```python
from build123d import *

# Parameters (mm, degrees)
SKETCH1_R                 = 10
BOSS_EXTRUDE2_DEPTH       = 35
SHELL1_T                  = -2.5
SHELL1_THICKNESS_2_FACE_R = 7.5
SHELL1_THICKNESS_2_DEPTH  = 27.5
SKETCH2_R                 = 1
BOSS_EXTRUDE3_DEPTH       = 40


with BuildPart() as part:
    # Sketch1 → Boss-Extrude2 (new body)
    with BuildSketch(Plane(origin=(0, 0, 0), x_dir=(1, 0, 0), z_dir=(0, 1, 0))):
        with Locations(Location((0, 0, 0), (0, 0, 270))):
            Circle(SKETCH1_R)
    extrude(amount=BOSS_EXTRUDE2_DEPTH)

    # Shell1
    shell1_openings = [part.faces().sort_by_distance(p)[0] for p in [
        (0, 35, 0),
    ]]
    offset(amount=SHELL1_T, openings=shell1_openings, kind=Kind.INTERSECTION)

    # Shell1 thickness 2 face (on inner face of the shell) → Shell1 thickness 2 (add)
    with BuildSketch(Plane(origin=(0, 2.5, 0), x_dir=(0, 0, -1), z_dir=(0, -1, 0))):
        Circle(SHELL1_THICKNESS_2_FACE_R)
    extrude(amount=-SHELL1_THICKNESS_2_DEPTH)

    # Sketch2 → Boss-Extrude3 (add)
    with BuildSketch(Plane(origin=(0, 30, 0), x_dir=(1, 0, 0), z_dir=(0, 1, 0))):
        with Locations(Location((0, 0, 0), (0, 0, 270))):
            Circle(SKETCH2_R)
    extrude(amount=BOSS_EXTRUDE3_DEPTH)


solid = part.part
```
Here's how the part is built. I have some questions about the finished solid (model axes, mm). A direction names the side the tool comes from. Coordinates: 2 decimals unless noted, no trailing zeros. Order: outer loops, then holes, each group sorted by start corner. A loop starts at its lowest first (then second) coordinate and runs counter-clockwise, first axis right, second up.
Item 1: Which directions (+Z, -Z, +X, -X, +Y, -Y) give clear straight access to the entire face, cutting with the end or side of a thin tool? Please do faces 1 (the face through (0, 70, 0)), 2 (the face through (-1, 50, 0)).
Response values:
face 1: +Z, -Z, +X, -X, +Y
face 2: +Y
Item 2: I need wall thicknesses on probe 1 along X at (y, z) = (32.45, 0); probe 2 along Z at (x, y) = (0.25, 34.5); probe 3 along Z at (x, y) = (0.5, 34). Which ranges of each line are inside material? Lowest first, please.
Response values:
probe 1: x = -10 to -7.5, -1 to 1, 7.5 to 10
probe 2: z = -10 to -7.5, -0.97 to 0.97, 7.5 to 10
probe 3: z = -9.99 to -7.48, -0.87 to 0.87, 7.48 to 9.99
Item 3: If we section it at D-D, the plane x = 5.5: List the corners of the cut face in (y, z) for me, then the cut area to 3 significant figures.
Response values:
outline: (0, -8.35) - (35, -8.35) - (35, -5.1) - (30, -5.1) - (30, 5.1) - (35, 5.1) - (35, 8.35) - (0, 8.35) - close
area: 534 mm2
Item 4: If we section it at A-A, the plane z = 0: List the corners of the cut face in (x, y) for me, then the cut area to 3 significant figures.
Response values:
outline: (-10, 0) - (10, 0) - (10, 35) - (7.5, 35) - (7.5, 30) - (1, 30) - (1, 70) - (-1, 70) - (-1, 30) - (-7.5, 30) - (-7.5, 35) - (-10, 35) - close
area: 705 mm2
Item 5: If we section it at C-C, the plane y = 5.5: List the corners of the cut face in (x, z) for me.
Response values:
outline: circle Ø20 at (0, 0)
Item 6: If we section it at B-B, the plane x = 0: List the corners of the cut face in (y, z) for me, then the cut area to 3 significant figures.
Response values:
outline: (0, -10) - (35, -10) - (35, -7.5) - (30, -7.5) - (30, -1) - (70, -1) - (70, 1) - (30, 1) - (30, 7.5) - (35, 7.5) - (35, 10) - (0, 10) - close
area: 705 mm2
Item 7: Thinking about a two-plate mould opening in Z: for faces 3 (the face through (-9.76, 17.26, -2.17)), 4 (the face through (0.33, 32.465, -7.493)), 5 (the face through (0, 0, 0)), which applies, pulls with the +Z half, pulls with the -Z half, needs draft (parallel to the pull), parting line crosses it, or undercut?
Response values:
face 3: parting line crosses it
face 4: undercut
face 5: needs draft
Item 8: I'm going to push flat-ended pins straight in: pin 1 Ø1 at (x, z) = (3.5, -6.5) entering from +Y; pin 2 Ø8 at (y, z) = (33.5, -5.5) entering from -X. Where does each tip first touch, or does it pass through?
Response values:
pin 1: stops at y = 35
pin 2: stops at x = -9.89
